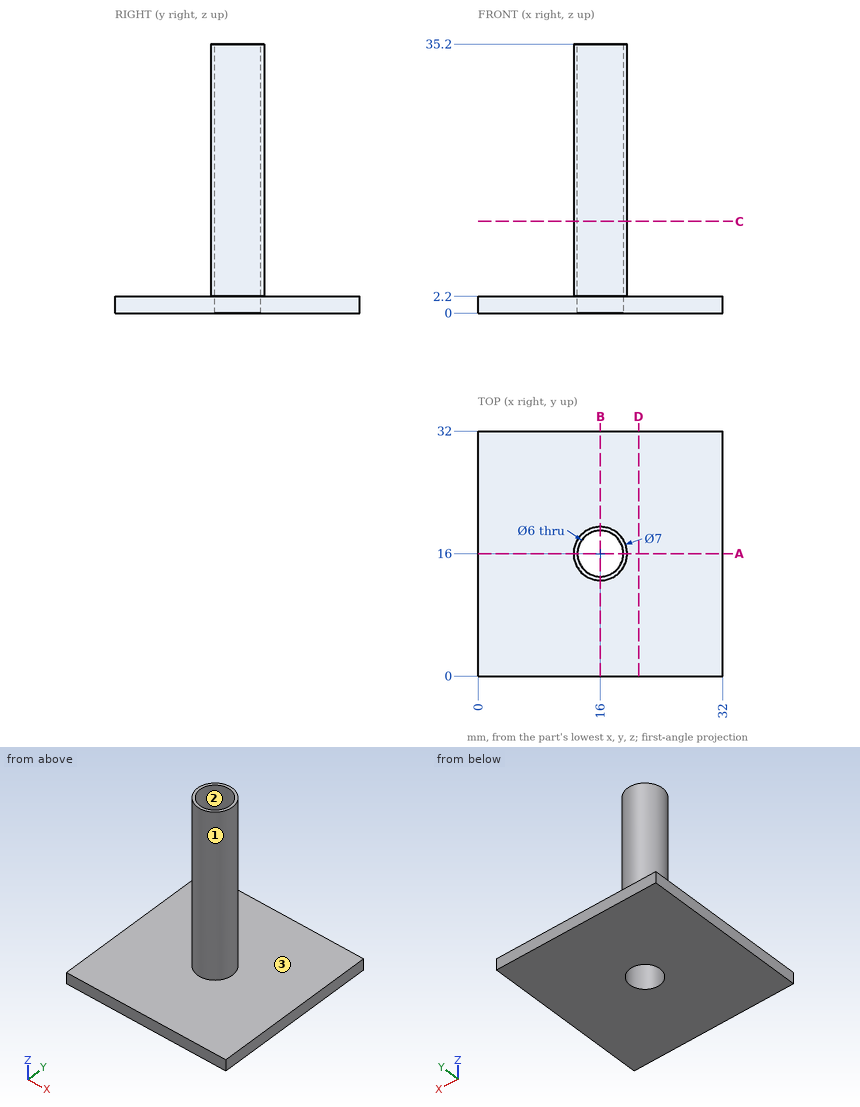
Check sheet for the drawn part. Datum: minimum x, y, z corner. Units: mm. Give positions to 0.01 mm unless a question says otherwise; leave off trailing zeros. Loops run counter-clockwise (first coordinate to the right, second up) from the corner with the lowest first, then second, coordinate; pieces in that order, holes last.
1) Sectioned sample at A-A, the plane y = 16. Enter the section's corners in (x, z), then the cut area to 3 significant figures.
2) Sectioned sample at D-D, the plane x = 21. Enter the section's corners in (y, z).
3) Thickness scan on line 1 along Y through (x, z) = (16, 15); line 2 along Z through (x, y) = (28, 22). Record the ranges inside material, lowest first.
4) Draft check along X on the marked faces 1, 2 and 3. Enter one of: pulls with the +X half, pulls with the -X half, needs draft (parallel to the pull), parting line crosses it, or undercut.
5) Depth check by flat-ended pin: pin 1 Ø1 at (x, y) = (11, 5) entering from +Z; pin 2 Ø6 at (x, z) = (20.5, 20.5) entering from -Y. Enter the tip coordinate at first touch or a pass-through.
6) Sectioned sample at C-C, the plane z = 12. Enter the section's corners in (x, y), then the cut area to 3 significant figures.
Answers:
1. outline: (0, 0) - (13, 0) - (13, 35.2) - (12.5, 35.2) - (12.5, 2.2) - (0, 2.2) - close; (19, 0) - (32, 0) - (32, 2.2) - (19.5, 2.2) - (19.5, 35.2) - (19, 35.2) - close
1. area: 90.2 mm2
2. outline: (0, 0) - (32, 0) - (32, 2.2) - (0, 2.2) - close
3. line 1: y = 12.5 to 13, 19 to 19.5
3. line 2: z = 0 to 2.2
4. face 1: parting line crosses it
4. face 2: undercut
4. face 3: needs draft
5. pin 1: stops at z = 2.2
5. pin 2: stops at y = 12.84
6. outline: circle Ø7 at (16, 16); hole circle Ø6 at (16, 16)
6. area: 10.2 mm2
